Read the model definition and answer for the solid it produces. Units are mm, in the model's axes. A direction names the side the tool comes from. Coordinates: 2 decimals unless noted, no trailing zeros. Write each loop counter-clockwise with the first axis right and the second up, starting at its lowest first coordinate (ties: lowest second). Pieces come first, ordered by that corner, then holes. Notation, with made-up numbers: (-29.75, 11) -> (-18.75, 11) arc R10 cw to (-18.75, 26) -> close; hole circle Ø2 at (0, 5.5). An arc over 180 degrees is marked (long way). Return JSON: item names as keys, results as strings.
from build123d import *

# Parameters (mm, degrees)
F0_W     = 35
F0_H     = 80
F1_DEPTH = 35
F2_SIZE2 = 25
F2_SIZE  = 75
F4_DEPTH = 35.001
F5_W     = 15
F5_H     = 25
F6_DEPTH = 10


with BuildPart() as f1:
    # F0 (on Top) → F1 (new body)
    with BuildSketch(Plane.XY):
        with Locations((0, -22.5)):
            Rectangle(F0_W, F0_H)
    extrude(amount=F1_DEPTH)

    # F2
    f2_edges = [f1.edges().sort_by_distance(p)[0] for p in [
        (0, 17.5, 35),
    ]]
    f2_side = f1.faces().sort_by_distance((0, -22.5, 35))[0]
    chamfer(f2_edges, length=F2_SIZE, length2=F2_SIZE2, reference=f2_side)

    # F3 (on face) → F4 (cut, through all)
    with BuildSketch(Plane(origin=(-17.5, 0, 0), x_dir=(0, -1, 0), z_dir=(-1, 0, 0))):
        Polygon((-7.5, 8.0628705664), (-7.5, 0), (52.5, 0), (52.5, 28.0628705664), align=None)
    extrude(amount=-F4_DEPTH, mode=Mode.SUBTRACT)

    # F5 (on face) → F6 (cut)
    with BuildSketch(Plane.XZ.offset(62.5)):
        with Locations((0, 12.5)):
            Rectangle(F5_W, F5_H)
    extrude(amount=-F6_DEPTH, mode=Mode.SUBTRACT)


solid = f1.part
1. The part is cut by section B-B (x = 1.5). Determine the outline of the cut face in (y, z), then the cut area to 3 significant figures.
Taken from the geometry:
{"outline": "(-62.5, 25) -> (-52.5, 25) -> (-52.5, 28.06) -> (7.5, 8.06) -> (7.5, 0) -> (17.5, 0) -> (17.5, 10) -> (-57.5, 35) -> (-62.5, 35) -> close", "area": "529 mm2"}
2. The part is cut by section D-D (y = -55.5). Determine the outline of the cut face in (x, z), then the cut area to 3 significant figures.
Taken from the geometry:
{"outline": "(-17.5, 0) -> (-7.5, 0) -> (-7.5, 25) -> (7.5, 25) -> (7.5, 0) -> (17.5, 0) -> (17.5, 34.33) -> (-17.5, 34.33) -> close", "area": "827 mm2"}
3. Consider L1, parallel to Y at x = -11.5, z = 3; L2, parallel to Y at x = 6, z = 3; L3, parallel to Z at x = 4, y = -22.5. Determine where each line is inside the solid, lowest interval first.
Taken from the geometry:
{"L1": "y = -62.5 to -52.5, 7.5 to 17.5", "L2": "y = 7.5 to 17.5", "L3": "z = 18.06 to 23.33"}
4. For a pull along Y with two mould halves and no side action, classify faces 1 (the face through (-8, -52.5, 14)), 2 (the face through (0, -58, 25)), 3 (the face through (-0.245, -22.92, 18.203)), 4 (the face through (8, -62.5, 17)) as +Y half, -Y half, draft (parallel to the pull), parting line (faces both ways), or undercut.
Taken from the geometry:
{"face 1": "undercut", "face 2": "draft", "face 3": "undercut", "face 4": "-Y half"}
5. The part is cut by section A-A (z = 5). Determine the outline of the cut face in (x, y), then the cut area to 3 significant figures.
Taken from the geometry:
{"outline": "(-17.5, -62.5) -> (-7.5, -62.5) -> (-7.5, -52.5) -> (-17.5, -52.5) -> close; (-17.5, 7.5) -> (17.5, 7.5) -> (17.5, 17.5) -> (-17.5, 17.5) -> close; (7.5, -62.5) -> (17.5, -62.5) -> (17.5, -52.5) -> (7.5, -52.5) -> close", "area": "550 mm2"}
6. A tool of negligible diameter and unlimited length cuts with its end or side. For faces 5 (the face through (0, 7.5, 4)), 6 (the face through (-0.245, -19.475, 22.325)), 7 (the face through (7.5, -58, 12)), from which of +Z, -Z, +X, -X, +Y, -Y can it reach the whole face along a straight path? Write none if from no direction.
Taken from the geometry:
{"face 5": "-Z, +X, -X", "face 6": "+Z, +X, -X, +Y", "face 7": "-Z, -Y"}
7. Flat-ended cylindrical pins translate along their axes: pin 1 Ø1 at (x, y) = (-2.5, -41) entering from -Z; pin 2 Ø6 at (x, y) = (-1.5, 6) entering from +Z; pin 3 Ø3 at (x, y) = (1.5, -59.5) entering from -Z. Find the tip coordinate at first contact, or state that the pin passes through.
Taken from the geometry:
{"pin 1": "stops at z = 24.06", "pin 2": "stops at z = 14.83", "pin 3": "stops at z = 25"}
8. The part is cut by section C-C (z = 31). Determine the outline of the cut face in (x, y), then the cut area to 3 significant figures.
Taken from the geometry:
{"outline": "(-17.5, -62.5) -> (17.5, -62.5) -> (17.5, -45.5) -> (-17.5, -45.5) -> close", "area": "595 mm2"}
